Design review of the part built by this model. Coordinates are the model's own, in mm. Coordinates: 2 decimals unless noted, no trailing zeros. Write each loop counter-clockwise with the first axis right and the second up, starting at its lowest first coordinate (ties: lowest second). Pieces come first, ordered by that corner, then holes.
Q1. To check wall thickness, follow probe 1 along X at (y, z) = (1.9, 25); probe 2 along Z at (x, y) = (-40.25, 2.7); probe 3 along X at (y, z) = (4.8, 24). State the ranges of each line that lie inside material, in increasing order.
Q2. Add section A-A, the plane z = 10. Give the boundary of the cut face in (x, y), plus the area to 3 significant figures.
Q3. Add section C-C, the plane z = -25. Give the boundary of the cut face in (x, y), plus the area to 3 significant figures.
Q4. Add section B-B, the plane x = 9.75. Give the boundary of the cut face in (y, z), plus the area to 3 significant figures.
from build123d import *

# Parameters (mm, degrees)
ESBO_O1_W                = 120
ESBO_O1_H                = 100
RESSALTO_EXTRUS_O1_DEPTH = 6
ESBO_O2_R                = 2.75
CORTE_EXTRUS_O1_DEPTH    = 79.33262411
FILETE1_R                = 8
ESBO_O3_R                = 2.5
CORTE_EXTRUS_O2_DEPTH    = 79.33262411


with BuildPart() as part:
    # Esboço1 → Ressalto-extrusão1 (new body)
    with BuildSketch(Plane(origin=(0, 0, 0), x_dir=(1, 0, 0), z_dir=(0, 1, 0))):
        Rectangle(ESBO_O1_W, ESBO_O1_H)
    extrude(amount=RESSALTO_EXTRUS_O1_DEPTH)

    # Esboço2 → Corte-extrusão1 (cut, through all)
    with BuildSketch(Plane(origin=(0, 6, 0), x_dir=(1, 0, 0), z_dir=(0, 1, 0))):
        with Locations(Location((9.75, 25, 0), (0, 0, 270))):
            Circle(ESBO_O2_R)
        with Locations(Location((40.25, 25, 0), (0, 0, 270))):
            Circle(ESBO_O2_R)
        with Locations(Location((9.75, -25, 0), (0, 0, 270))):
            Circle(ESBO_O2_R)
        with Locations(Location((40.25, -25, 0), (0, 0, 270))):
            Circle(ESBO_O2_R)
        with Locations(Location((-40.25, -25, 0), (0, 0, 90))):
            Circle(ESBO_O2_R)
        with Locations(Location((-9.75, -25, 0), (0, 0, 90))):
            Circle(ESBO_O2_R)
        with Locations(Location((-40.25, 25, 0), (0, 0, 90))):
            Circle(ESBO_O2_R)
        with Locations(Location((-9.75, 25, 0), (0, 0, 90))):
            Circle(ESBO_O2_R)
    extrude(amount=-CORTE_EXTRUS_O1_DEPTH, mode=Mode.SUBTRACT)

    # Filete1
    filete1_edges = [part.edges().sort_by_distance(p)[0] for p in [
        (60, 3, 50),
        (-60, 3, 50),
        (-60, 3, -50),
        (60, 3, -50),
    ]]
    fillet(filete1_edges, radius=FILETE1_R)

    # Esboço3 → Corte-extrusão2 (cut, through all)
    with BuildSketch(Plane(origin=(0, 6, 0), x_dir=(1, 0, 0), z_dir=(0, 1, 0))):
        with Locations(Location((52, 10, 0), (0, 0, 270))):
            Circle(ESBO_O3_R)
        with Locations(Location((52, -10, 0), (0, 0, 270))):
            Circle(ESBO_O3_R)
    extrude(amount=-CORTE_EXTRUS_O2_DEPTH, mode=Mode.SUBTRACT)


solid = part.part
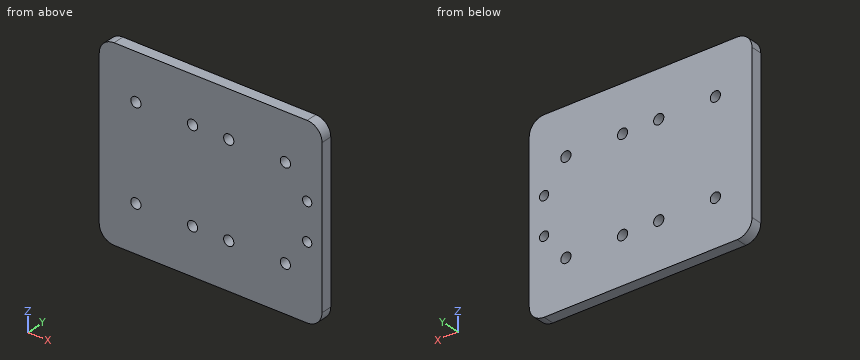
Here are the results:
1. probe 1: x = -60 to -43, -37.5 to -12.5, -7 to 7, 12.5 to 37.5, 43 to 60
1. probe 2: z = -50 to -27.75, -22.25 to 22.25, 27.75 to 50
1. probe 3: x = -60 to -42.81, -37.69 to -12.31, -7.19 to 7.19, 12.31 to 37.69, 42.81 to 60
2. outline: (-60, 0) - (49.5, 0) - (49.5, 6) - (-60, 6) - close; (54.5, 0) - (60, 0) - (60, 6) - (54.5, 6) - close
2. area: 690 mm2
3. outline: (-60, 0) - (-43, 0) - (-43, 6) - (-60, 6) - close; (-37.5, 0) - (-12.5, 0) - (-12.5, 6) - (-37.5, 6) - close; (-7, 0) - (7, 0) - (7, 6) - (-7, 6) - close; (12.5, 0) - (37.5, 0) - (37.5, 6) - (12.5, 6) - close; (43, 0) - (60, 0) - (60, 6) - (43, 6) - close
3. area: 588 mm2
4. outline: (0, -50) - (6, -50) - (6, -27.75) - (0, -27.75) - close; (0, -22.25) - (6, -22.25) - (6, 22.25) - (0, 22.25) - close; (0, 27.75) - (6, 27.75) - (6, 50) - (0, 50) - close
4. area: 534 mm2
